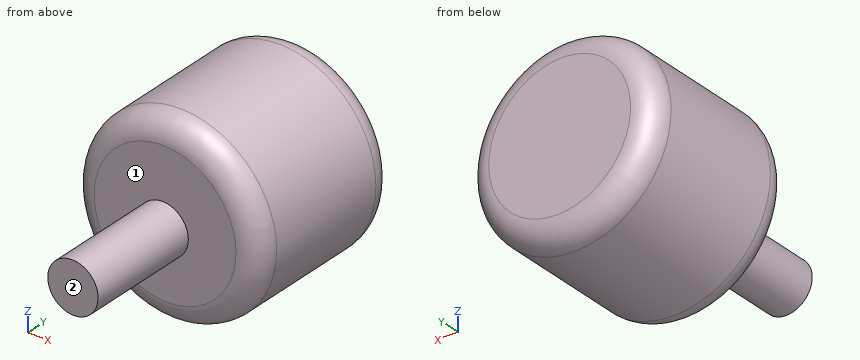
```python
from build123d import *

# Parameters (mm, degrees)
F0_R     = 20.987211
F1_DEPTH = 38.1
F2_R     = 5.08
F3_R     = 5.64864
F4_DEPTH = 25.4


with BuildPart() as f1:
    # F0 (on Front) → F1 (new body)
    with BuildSketch(Plane.XZ):
        with Locations((-26.213065, 26.794255)):
            Circle(F0_R)
    extrude(amount=-F1_DEPTH)

    # F2
    f2_edges = [f1.edges().sort_by_distance(p)[0] for p in [
        (-47.200276, 0, 26.794255),
        (-5.225854, 19.05, 26.794255),
        (-47.200276, 38.1, 26.794255),
    ]]
    fillet(f2_edges, radius=F2_R)

    # F3 (on Front) → F4 (join)
    with BuildSketch(Plane.XZ):
        with Locations((-26.644299, 25.517916)):
            Circle(F3_R)
    extrude(amount=F4_DEPTH)


solid = f1.part
```
CAD build for the part. Positions are in the model's coordinates, mm. Face numbers are marked on the shaded views. A direction names the side the tool comes from. Coordinates: 2 decimals unless noted, no trailing zeros. Loops run counter-clockwise (first coordinate to the right, second up) from the corner with the lowest first, then second, coordinate; pieces in that order, holes last. Notation, with made-up numbers: (10, 49) - (35, 49) arc R16 cw to (35, 72) - close; hole circle Ø8 at (4, 40.5). An arc over 180 degrees is marked (long way). Return JSON: item names as keys, results as strings.
1. Band-saw the part on B-B (y = -18.5). Give the cut face in (x, z), and give its area (3 significant figures).
Result:
{"outline": "circle Ø11.3 at (-26.64, 25.52)", "area": "100 mm2"}
2. Drop flat-ended pins along their axis: pin 1 (8 mm diameter, centred on x = -18.5, y = -11.5, fed in from -Z); pin 2 (1.5 mm diameter, centred on x = -29.5, z = 41.5, fed in from -Y); pin 3 (12 mm diameter, centred on x = -24, y = -10, fed in from +Z). Give the stop position or say it passes through.
Result:
{"pin 1": "stops at z = 21.68", "pin 2": "stops at y = 0", "pin 3": "stops at z = 31.17"}
3. Probe L1, parallel to Y at x = -35.5, z = 26; L2, parallel to X at y = 26.5, z = 27; L3, parallel to Z at x = -27, y = -11.5. List the from-to ranges inside material, lowest first. Write a range as from..to.
Result:
{"L1": "y = 0..38.1", "L2": "x = -47.2..-5.23", "L3": "z = 19.88..31.16"}
4. Band-saw the part on A-A (y = 1). Give the cut face in (x, z), and give its area (3 significant figures).
Result:
{"outline": "circle Ø37.87 at (-26.21, 26.79)", "area": "1,130 mm2"}
5. 3-axis set-ups, long thin cutter, end or side, ignore diameter. For the marked faces 1 and 2: which of +Z, -Z, +X, -X, +Y, -Y reach the whole face in a straight line?
Result:
{"face 1": "-Y", "face 2": "+Z, -Z, +X, -X, -Y"}
